For this review, take the finished solid that the model builds, in its own axes (mm). A direction names the side the tool comes from. Give positions to 0.01 mm unless a question says otherwise; leave off trailing zeros. Loops run counter-clockwise (first coordinate to the right, second up) from the corner with the lowest first, then second, coordinate; pieces in that order, holes last. Notation, with made-up numbers: (81, -12.5) - (124, -12.5) arc R35 cw to (124, 25.5) - close; hole circle Ø7 at (-23, 60.5). An arc over 180 degrees is marked (long way). Put each result on its own line as item: value.
from build123d import *

# Parameters (mm, degrees)
F0_W        = 12
F0_H        = 10
F1_DEPTH    = 18
F2_T1_DEPTH = 56.7298334621
F2_T3_DEPTH = 58


# Not quite as in the source:
# - a fillet or chamfer that OpenCascade refuses, or shapes differently, is made with other operations: its cross-section is extruded or revolved along the edge and cut away or added


with BuildPart() as f1:
    # F0 (on Top) → F1 (new body)
    with BuildSketch(Plane.XY):
        with BuildLine():
            ThreePointArc((14.4251908534, 16.4576590359), (22.1711575458, 22.4576590359), (29.9171242382, 16.4576590359))
            Line((29.9171242382, 16.4576590359), (34.1711575458, 16.4576590359))
            Line((34.1711575458, 16.4576590359), (34.1711575458, 26.4576590359))
            Line((34.1711575458, 26.4576590359), (23.6711575458, 26.4576590359))
            ThreePointArc((23.6711575458, 26.4576590359), (22.1711575458, 25.9576590359), (20.6711575458, 26.4576590359))
            Line((20.6711575458, 26.4576590359), (10.8711575458, 26.4576590359))
            Line((10.8711575458, 26.4576590359), (10.8711575458, 16.4576590359))
            Line((10.8711575458, 16.4576590359), (14.4251908534, 16.4576590359))
        make_face()
        with BuildLine():
            Line((34.1711575458, 12.4576590359), (29.9171242382, 12.4576590359))
            ThreePointArc((29.9171242382, 12.4576590359), (22.1711575458, 6.4576590359), (14.4251908534, 12.4576590359))
            Line((14.4251908534, 12.4576590359), (10.8711575458, 12.4576590359))
            Line((10.8711575458, 12.4576590359), (10.8711575458, 2.4576590359))
            Line((10.8711575458, 2.4576590359), (20.6711575458, 2.4576590359))
            ThreePointArc((20.6711575458, 2.4576590359), (22.1711575458, 2.9576590359), (23.6711575458, 2.4576590359))
            Line((23.6711575458, 2.4576590359), (34.1711575458, 2.4576590359))
            Line((34.1711575458, 2.4576590359), (34.1711575458, 12.4576590359))
        make_face()
        with BuildLine():
            ThreePointArc((14.4251908534, 12.4576590359), (14.1711575458, 14.4576590359), (14.4251908534, 16.4576590359))
            Line((14.4251908534, 16.4576590359), (10.8711575458, 16.4576590359))
            Line((10.8711575458, 16.4576590359), (10.8711575458, 12.4576590359))
            Line((10.8711575458, 12.4576590359), (14.4251908534, 12.4576590359))
        make_face()
        with Locations((40.1711575458, 21.4576590359)):
            Rectangle(F0_W, F0_H)
        with Locations((40.1711575458, 7.4576590359)):
            Rectangle(F0_W, F0_H)
        with BuildLine():
            Line((23.6711575458, 26.4576590359), (34.1711575458, 26.4576590359))
            Line((34.1711575458, 26.4576590359), (34.1711575458, 32.4576590359))
            Line((34.1711575458, 32.4576590359), (10.8711575458, 32.4576590359))
            Line((10.8711575458, 32.4576590359), (10.8711575458, 26.4576590359))
            Line((10.8711575458, 26.4576590359), (20.6711575458, 26.4576590359))
            ThreePointArc((20.6711575458, 26.4576590359), (21.0531235571, 30.6937270134), (24.6711575458, 28.4576590359))
            ThreePointArc((24.6711575458, 28.4576590359), (24.4072255233, 27.3396250472), (23.6711575458, 26.4576590359))
        make_face()
        with BuildLine():
            Line((34.1711575458, -3.5423409641), (34.1711575458, 2.4576590359))
            Line((34.1711575458, 2.4576590359), (23.6711575458, 2.4576590359))
            ThreePointArc((23.6711575458, 2.4576590359), (24.4072255233, 1.5756930247), (24.6711575458, 0.4576590359))
            ThreePointArc((24.6711575458, 0.4576590359), (21.0531235571, -1.7784089416), (20.6711575458, 2.4576590359))
            Line((20.6711575458, 2.4576590359), (10.8711575458, 2.4576590359))
            Line((10.8711575458, 2.4576590359), (10.8711575458, -3.5423409641))
            Line((10.8711575458, -3.5423409641), (34.1711575458, -3.5423409641))
        make_face()
    extrude(amount=F1_DEPTH)

    # F2: fillet of radius 8 on 4 edges, made by hand

    # F2_s2 → F2_t1 (cut)
    with BuildSketch(Plane.XY.offset(-19.364916731)):
        with BuildLine():
            ThreePointArc((34.1711575458, 26.4576590359), (31.324170339, 30.7822143563), (26.4251908534, 32.4576590359))
            Line((26.4251908534, 32.4576590359), (34.1711575458, 32.4576590359))
            Line((34.1711575458, 32.4576590359), (34.1711575458, 26.4576590359))
        make_face()
        with BuildLine():
            ThreePointArc((26.4251908534, -3.5423409641), (31.324170339, -1.8668962844), (34.1711575458, 2.4576590359))
            Line((34.1711575458, 2.4576590359), (34.1711575458, -3.5423409641))
            Line((34.1711575458, -3.5423409641), (26.4251908534, -3.5423409641))
        make_face()
    extrude(amount=F2_T1_DEPTH, mode=Mode.SUBTRACT)

    # F2_s4 → F2_t3 (cut)
    with BuildSketch(Plane.XY.offset(-20)):
        with BuildLine():
            ThreePointArc((10.8711575458, 4.4576590359), (13.2143032963, -1.1991952136), (18.8711575458, -3.5423409641))
            Line((18.8711575458, -3.5423409641), (10.8711575458, -3.5423409641))
            Line((10.8711575458, -3.5423409641), (10.8711575458, 4.4576590359))
        make_face()
        with BuildLine():
            ThreePointArc((18.8711575458, 32.4576590359), (13.2143032963, 30.1145132854), (10.8711575458, 24.4576590359))
            Line((10.8711575458, 24.4576590359), (10.8711575458, 32.4576590359))
            Line((10.8711575458, 32.4576590359), (18.8711575458, 32.4576590359))
        make_face()
    extrude(amount=F2_T3_DEPTH, mode=Mode.SUBTRACT)


solid = f1.part
1) Draft analysis for pull direction Y (two halves, no side actions). For faces 4 (the face through (40, 2.458, 9)), 5 (the face through (31.38, 30.74, 8.87)), 6 (the face through (38, 12.458, 9)), state which applies: pulls with the +Y half, pulls with the -Y half, needs draft (parallel to the pull), parting line crosses it, or undercut.
Geometry check:
face 4: pulls with the -Y half
face 5: pulls with the +Y half
face 6: undercut
2) Take a section at B-B on y = 10. State the section outline as (x, z) points, and give its area (3 significant figures).
Geometry check:
outline: (10.87, 0) - (15.53, 0) - (15.53, 18) - (10.87, 18) - close; (28.81, 0) - (46.17, 0) - (46.17, 18) - (28.81, 18) - close
area: 396 mm²
3) Take a section at A-A on x = 35. State the section outline as (y, z) points, and give its area (3 significant figures).
Geometry check:
outline: (2.46, 0) - (12.46, 0) - (12.46, 18) - (2.46, 18) - close; (16.46, 0) - (26.46, 0) - (26.46, 18) - (16.46, 18) - close
area: 360 mm²
4) Insertion check: pin 1 Ø8 at (x, y) = (21.5, 11.5) entering from +Z; pin 2 Ø9.5 at (x, z) = (42, 13) entering from -Y; pin 3 Ø9.5 at (x, z) = (39.5, 11.5) entering from +Y. Each pin has a flat end and moves straight along its axis. Give the tip position at first contact, or say it passes through.
Geometry check:
pin 1: passes through
pin 2: stops at y = 2.46
pin 3: stops at y = 26.46
5) Take a section at C-C on z = 3.5. State the section outline as (x, y) points, and give its area (3 significant figures).
Geometry check:
outline: (10.87, 4.46) arc R8 ccw to (18.87, -3.54) - (26.43, -3.54) arc R8 ccw to (34.17, 2.46) - (46.17, 2.46) - (46.17, 12.46) - (29.92, 12.46) arc R8 cw (long way) to (29.92, 16.46) - (46.17, 16.46) - (46.17, 26.46) - (34.17, 26.46) arc R8 ccw to (26.43, 32.46) - (18.87, 32.46) arc R8 ccw to (10.87, 24.46) - close; hole circle Ø5 at (22.17, 0.46); hole circle Ø5 at (22.17, 28.46)
area: 771 mm²
6) Wall thickness on line 1 (Y direction, x = 40.5, z = 13.75); line 2 (Y direction, x = 23.5, z = 14.75); line 3 (X direction, y = 21.5, z = 9.5): over which ranges is each line inside the solid? List them lowest first.
Geometry check:
line 1: y = 2.46 to 12.46, 16.46 to 26.46
line 2: y = -3.54 to -1.66, 2.58 to 6.57, 22.35 to 26.34, 30.58 to 32.46
line 3: x = 10.87 to 18.38, 25.97 to 46.17
7) For faces 1 (the face through (38, 16.458, 9)), 2 (the face through (32, 11, 0)), 3 (the face through (40, 26.458, 9)), list the 3-axis set-ups (+Z, -Z, +X, -X, +Y, -Y) from which the entire face can be reached by the end or side of a thin tool; tool diameter is ignored.
Geometry check:
face 1: +Z, -Z, +X
face 2: -Z, +X, -X, +Y, -Y
face 3: +Z, -Z, +X, +Y
